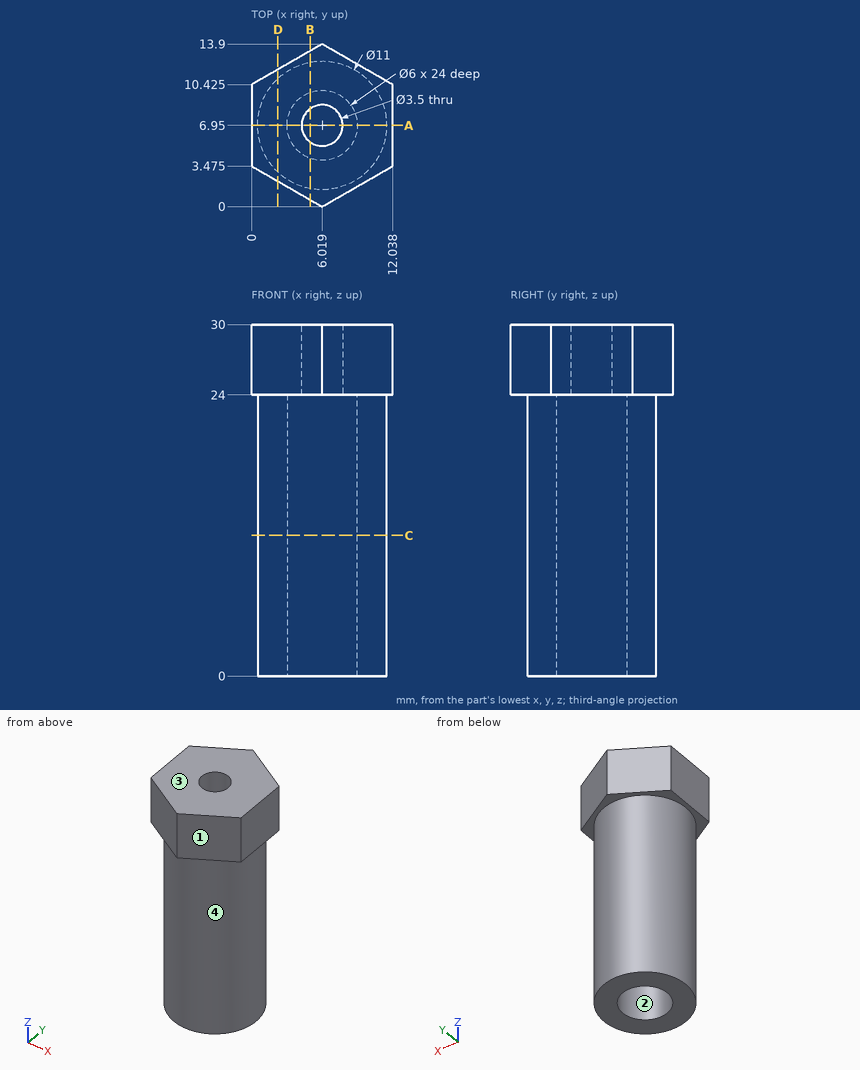
Could you check a few things on this drawing? It's one solid part, dimensions in mm from its lowest x, y, z. Give positions to 0.01 mm unless a question says otherwise; leave off trailing zeros. Order: outer loops, then holes, each group sorted by start corner. A loop starts at its lowest first (then second) coordinate and runs counter-clockwise, first axis right, second up. Notation, with made-up numbers: (29.5, -19) - (33.5, -19) arc R18 cw to (33.5, -2) - close; hole circle Ø5 at (46.5, -26.75). An arc over 180 degrees is marked (long way). Answer as a JSON object with one key per item and string values. Group by question number.
Item 1: If we section it at D-D on x = 2.25: Please give me the cut outline in (y, z).
Item 2: If we mould it in two halves opening along X, with no side actions, what happens to the marked faces 1, 2, 3 and 4? For each: pulls with the +X half, pulls with the -X half, needs draft (parallel to the pull), parting line crosses it, or undercut.
Item 3: If we section it at C-C on z = 12: Please give me the cut outline in (x, y).
Item 4: If we section it at B-B on x = 5: Please give me the cut outline in (y, z) (1 decimal).
Item 5: Please list where these lines run through material, in increasing order: probe 1 along X at (y, z) = (7, 27); probe 2 along X at (y, z) = (9.25, 12) (1 decimal); probe 3 along Z at (x, y) = (6, 4.5).
Item 6: If we section it at A-A on y = 6.95: Please give me the cut outline in (x, z).
Item 7: For P1, Ø1, axis at y = 8, z = 4.5, coming from the +X side; P2, Ø6, axis at x = 9, z = 11, coming from the +Y side; P3, Ø6.5, axis at x = 4.5, y = 7, coming from the -Z side; P4, Ø5, axis at y = 3, z = 17, coming from the +X side, each with a flat end and sliding along its axis, tell me the tip position at first contact or that it passes through.
Result set:
{
 "1": {"outline": "(2.18, 24) - (2.94, 24) - (2.94, 0) - (10.96, 0) - (10.96, 24) - (11.72, 24) - (11.72, 30) - (2.18, 30) - close"},
 "2": {"face 1": "pulls with the +X half", "face 2": "undercut", "face 3": "needs draft", "face 4": "parting line crosses it"},
 "3": {"outline": "circle Ø11 at (6.02, 6.95); hole circle Ø6 at (6.02, 6.95)"},
 "4": {"outline": "(0.6, 24) - (1.5, 24) - (1.5, 0) - (4.1, 0) - (4.1, 24) - (5.5, 24) - (5.5, 30) - (0.6, 30) - close; (8.4, 24) - (9.8, 24) - (9.8, 0) - (12.4, 0) - (12.4, 24) - (13.3, 24) - (13.3, 30) - (8.4, 30) - close"},
 "5": {"probe 1": "0 to 4.27, 7.77 to 12.04", "probe 2": "1 to 4.1, 7.9 to 11", "probe 3": "24 to 30"},
 "6": {"outline": "(0, 24) - (0.52, 24) - (0.52, 0) - (3.02, 0) - (3.02, 24) - (4.27, 24) - (4.27, 30) - (0, 30) - close; (7.77, 24) - (9.02, 24) - (9.02, 0) - (11.52, 0) - (11.52, 24) - (12.04, 24) - (12.04, 30) - (7.77, 30) - close"},
 "7": {"P1": "x = 11.49", "P2": "y = 12.45", "P3": "z = 0", "P4": "x = 11.32"}
}
